Input: part model. Units: mm. Frame: model coordinates. Face numbers are marked on the shaded views. A direction names the side the tool comes from. Coordinates: 2 decimals unless noted, no trailing zeros. Write each loop counter-clockwise with the first axis right and the second up, starting at its lowest first coordinate (ties: lowest second). Pieces come first, ordered by that corner, then holes.
1) Section query A-A (y = 10). Output: boundary loops of the cut face in (x, z), then the cut area to 3 significant figures.
2) Pin query (flat end, axial travel): pin 1 Ø2 at (y, z) = (0.5, 2) entering from -X; pin 2 Ø1.5 at (y, z) = (-33, 7) entering from -X; pin 3 Ø2.5 at (y, z) = (-21.5, 2) entering from -X. Return the tip coordinate at first contact, or that it passes through.
3) Section query D-D (y = 33). Output: boundary loops of the cut face in (x, z).
4) Section query B-B (x = 6). Output: boundary loops of the cut face in (y, z).
5) Line query: L1, parallel to Y at x = -2.5, z = 1.5; L2, parallel to Y at x = -2, z = 5.75; L3, parallel to X at y = 38, z = 6. Output: solid intervals per line, ascending.
6) Draft query along X for the marked faces 1, 2 and 3. Return one class per face: pulls with the +X half, pulls with the -X half, needs draft (parallel to the pull), parting line crosses it, or undercut.
7) Section query C-C (z = 5.75). Output: boundary loops of the cut face in (x, y), then the cut area to 3 significant figures.
8) Set-up query: the marked faces 4 and 5. Return all of +Z, -Z, +X, -X, +Y, -Y with unobstructed straight access to the full face (end or side cutting, diameter ignored); none if empty.
from build123d import *

# Parameters (mm, degrees)
F0_R     = 11.0109
F1_DEPTH = 7.747


with BuildPart() as f1:
    # F0 (on Top) → F1 (new body)
    with BuildSketch(Plane.XY):
        with BuildLine():
            Line((20.392826, -13.514568), (8.224028, 14.635976))
            ThreePointArc((8.224028, 14.635976), (14.048919, 32.063751), (0, 43.907929))
            Line((0, 43.907929), (-20.211583, 43.907929))
            Line((-20.211583, 43.907929), (-20.392826, 13.514568))
            Line((-20.392826, 13.514568), (-8.224028, -14.635976))
            ThreePointArc((-8.224028, -14.635976), (-14.048919, -32.063751), (0, -43.907929))
            Line((0, -43.907929), (20.211583, -43.907929))
            Line((20.211583, -43.907929), (20.392826, -13.514568))
        make_face()
        with Locations((0, -28.3718)):
            Circle(F0_R, mode=Mode.SUBTRACT)
        with BuildLine():
            Line((16.587436, -13.514568), (16.587436, -38.889877))
            Line((16.587436, -38.889877), (10.177375, -38.851653))
            ThreePointArc((10.177375, -38.851653), (13.6719, -28.159103), (10.177375, -17.466553))
            Line((10.177375, -17.466553), (9.983805, -13.514568))
            Line((9.983805, -13.514568), (16.587436, -13.514568))
        make_face(mode=Mode.SUBTRACT)
        with BuildLine():
            Line((-16.587436, 13.514568), (-16.587436, 38.889877))
            Line((-16.587436, 38.889877), (-10.177375, 38.851653))
            ThreePointArc((-10.177375, 38.851653), (-13.6719, 28.159103), (-10.177375, 17.466553))
            Line((-10.177375, 17.466553), (-9.983805, 13.514568))
            Line((-9.983805, 13.514568), (-16.587436, 13.514568))
        make_face(mode=Mode.SUBTRACT)
        Circle(F0_R, mode=Mode.SUBTRACT)
        with Locations((0, 28.3718)):
            Circle(F0_R, mode=Mode.SUBTRACT)
    extrude(amount=F1_DEPTH)


solid = f1.part
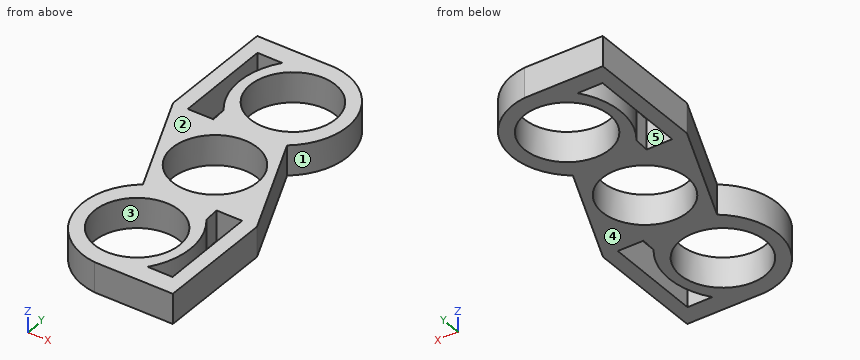
Answer:
1. outline: (-18.87, 0) - (-4.61, 0) - (-4.61, 7.75) - (-18.87, 7.75) - close; (4.61, 0) - (10.23, 0) - (10.23, 7.75) - (4.61, 7.75) - close
1. area: 154 mm2
2. pin 1: stops at x = -15.2
2. pin 2: stops at x = -14
2. pin 3: stops at x = -13.91
3. outline: (-20.28, 0) - (-16.59, 0) - (-16.59, 7.75) - (-20.28, 7.75) - close; (-13.01, 0) - (-9.99, 0) - (-9.99, 7.75) - (-13.01, 7.75) - close; (9.99, 0) - (13.76, 0) - (13.76, 7.75) - (9.99, 7.75) - close
4. outline: (-43.91, 0) - (-37.6, 0) - (-37.6, 7.75) - (-43.91, 7.75) - close; (-19.14, 0) - (-9.23, 0) - (-9.23, 7.75) - (-19.14, 7.75) - close; (9.23, 0) - (19.14, 0) - (19.14, 7.75) - (9.23, 7.75) - close; (37.6, 0) - (42.07, 0) - (42.07, 7.75) - (37.6, 7.75) - close
5. L1: y = -43.45 to -39.1, -17.65 to -10.72, 10.72 to 17.65, 39.1 to 43.91
5. L2: y = -43.57 to -39.2, -17.54 to -10.83, 10.83 to 17.54, 39.2 to 43.91
5. L3: x = -20.25 to -16.59, -10.76 to -5.34, 5.34 to 10.96
6. face 1: pulls with the +X half
6. face 2: needs draft
6. face 3: undercut
7. outline: (-20.39, 13.51) - (-8.22, -14.64) arc R16.36 ccw to (0, -43.91) - (20.21, -43.91) - (20.39, -13.51) - (8.22, 14.64) arc R16.36 ccw to (0, 43.91) - (-20.21, 43.91) - close; hole (-16.59, 13.51) - (-9.98, 13.51) - (-10.18, 17.47) arc R18.11 cw to (-10.18, 38.85) - (-16.59, 38.89) - close; hole circle Ø22.02 at (0, -28.37); hole circle Ø22.02 at (0, 0); hole circle Ø22.02 at (0, 28.37); hole (9.98, -13.51) - (10.18, -17.47) arc R18.11 cw to (10.18, -38.85) - (16.59, -38.89) - (16.59, -13.51) - close
7. area: 1,370 mm2
8. face 4: -Z, +X, -X, +Y, -Y
8. face 5: +Z, -Z
